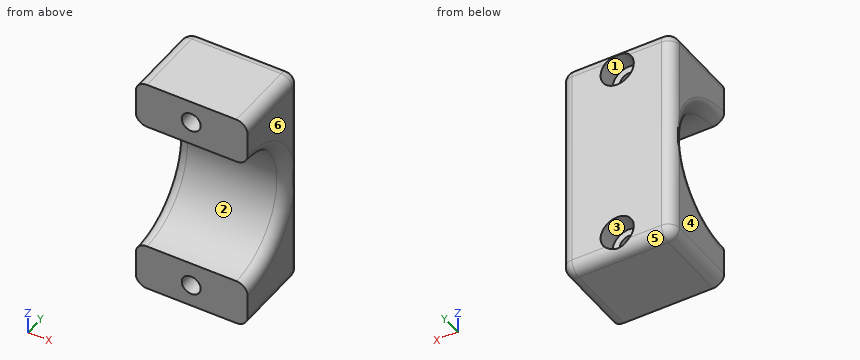
from build123d import *

# Parameters (mm, degrees)
SKETCH1_W                                      = 50.8
SKETCH1_H                                      = 19.05
BOSS_EXTRUDE1_DEPTH                            = 25.4
SKETCH2_R                                      = 14.9225
CUT_EXTRUDE1_DEPTH                             = 60.905780189
CBORE_FOR_6_BUTTON_HEAD_CAP_SCREW1_D           = 4.3053
CBORE_FOR_6_BUTTON_HEAD_CAP_SCREW1_CBORE_D     = 7.54126
CBORE_FOR_6_BUTTON_HEAD_CAP_SCREW1_CBORE_DEPTH = 4.3942
FILLET1_R                                      = 2.54


with BuildPart() as part:
    # Sketch1 → Boss-Extrude1 (new body)
    with BuildSketch(Plane(origin=(0, 0, 0), x_dir=(0, 0, -1), z_dir=(1, 0, 0))):
        with Locations((25.4, 9.525)):
            Rectangle(SKETCH1_W, SKETCH1_H)
    extrude(amount=BOSS_EXTRUDE1_DEPTH)

    # Sketch2 → Cut-Extrude1 (cut, through all)
    with BuildSketch(Plane(origin=(25.4, 0, 0), x_dir=(0, 0, -1), z_dir=(1, 0, 0))):
        with Locations((25.4, 0)):
            Circle(SKETCH2_R)
    extrude(amount=-CUT_EXTRUDE1_DEPTH, mode=Mode.SUBTRACT)

    # CBORE for #6 Button Head Cap Screw1 (through all)
    with Locations(Plane(origin=(0, 19.05, 0), x_dir=(1, 0, 0), z_dir=(0, 1, 0))):
        with Locations((12.594620829, 5.08), (12.594620829, 45.72)):
            CounterBoreHole(CBORE_FOR_6_BUTTON_HEAD_CAP_SCREW1_D / 2, CBORE_FOR_6_BUTTON_HEAD_CAP_SCREW1_CBORE_D / 2, CBORE_FOR_6_BUTTON_HEAD_CAP_SCREW1_CBORE_DEPTH)

    # Fillet1
    # the kernel refuses this fillet: 2.54 mm, written as the material it takes off along each edge
    with BuildSketch(Plane(origin=(22.86, 16.51, -48.26), x_dir=(0, 1, 0), z_dir=(1, 0, 0))) as fillet1_piece_1_section:
        Polygon((0, 0), (FILLET1_R, 0), (FILLET1_R, -FILLET1_R), (0, -FILLET1_R), align=None)
    fillet1_piece_1 = extrude(amount=FILLET1_R, mode=Mode.PRIVATE)
    fillet1_piece_1 = fillet1_piece_1 - Plane(origin=(22.86, 16.51, -48.26), x_dir=(0, -0.7071067811865475, 0.7071067811865475), z_dir=(1, 0, 0)) * Sphere(FILLET1_R, mode=Mode.PRIVATE)
    add(fillet1_piece_1, mode=Mode.SUBTRACT)
    with BuildSketch(Plane(origin=(22.86, 16.51, -2.54), x_dir=(1, 0, 0), z_dir=(0, 0, 1))) as fillet1_piece_2_section:
        Polygon((0, 0), (FILLET1_R, 0), (FILLET1_R, FILLET1_R), (0, FILLET1_R), align=None)
    fillet1_piece_2 = extrude(amount=FILLET1_R, mode=Mode.PRIVATE)
    fillet1_piece_2 = fillet1_piece_2 - Plane(origin=(22.86, 16.51, -2.54), x_dir=(-0.7071067811865475, -0.7071067811865475, 0), z_dir=(0, 0, 1)) * Sphere(FILLET1_R, mode=Mode.PRIVATE)
    add(fillet1_piece_2, mode=Mode.SUBTRACT)
    with BuildSketch(Plane(origin=(2.54, 16.51, -48.26), x_dir=(0, 1, 0), z_dir=(-1, 0, 0))) as fillet1_piece_3_section:
        Polygon((0, 0), (FILLET1_R, 0), (FILLET1_R, FILLET1_R), (0, FILLET1_R), align=None)
    fillet1_piece_3 = extrude(amount=FILLET1_R, mode=Mode.PRIVATE)
    fillet1_piece_3 = fillet1_piece_3 - Plane(origin=(2.54, 16.51, -48.26), x_dir=(0, -0.7071067811865475, 0.7071067811865475), z_dir=(-1, 0, 0)) * Sphere(FILLET1_R, mode=Mode.PRIVATE)
    add(fillet1_piece_3, mode=Mode.SUBTRACT)
    with BuildSketch(Plane(origin=(2.54, 16.51, -2.54), x_dir=(0, 0, 1), z_dir=(-1, 0, 0))) as fillet1_piece_4_section:
        Polygon((0, 0), (FILLET1_R, 0), (FILLET1_R, FILLET1_R), (0, FILLET1_R), align=None)
    fillet1_piece_4 = extrude(amount=FILLET1_R, mode=Mode.PRIVATE)
    fillet1_piece_4 = fillet1_piece_4 - Plane(origin=(2.54, 16.51, -2.54), x_dir=(0, -0.7071067811865475, -0.7071067811865475), z_dir=(-1, 0, 0)) * Sphere(FILLET1_R, mode=Mode.PRIVATE)
    add(fillet1_piece_4, mode=Mode.SUBTRACT)
    with BuildSketch(Plane(origin=(25.4, -6.35, -50.8), x_dir=(0, 0, 1), z_dir=(0, 1, 0))) as fillet1_piece_5:
        with BuildLine():
            CenterArc((FILLET1_R, -FILLET1_R), FILLET1_R, 90, 90)
            Line((0, -FILLET1_R), (0, 0))
            Line((0, 0), (FILLET1_R, 0))
        make_face()
    extrude(amount=22.86, mode=Mode.SUBTRACT)
    with BuildSketch(Plane(origin=(25.4, 19.05, -48.26), x_dir=(0, -1, 0), z_dir=(0, 0, 1))) as fillet1_piece_6:
        with BuildLine():
            CenterArc((FILLET1_R, -FILLET1_R), FILLET1_R, 90, 90)
            Line((0, -FILLET1_R), (0, 0))
            Line((0, 0), (FILLET1_R, 0))
        make_face()
    extrude(amount=45.72, mode=Mode.SUBTRACT)
    with BuildSketch(Plane(origin=(25.4, 0, -25.4), x_dir=(0, -0.413428527977308, -0.9105365738148667), z_dir=(0, -0.9105365738148667, 0.413428527977308))) as fillet1_piece_7:
        with BuildLine():
            CenterArc((14.9225 + FILLET1_R, -FILLET1_R), FILLET1_R, 90, 90)
            Line((14.9225 + FILLET1_R, 0), (14.9225, 0))
            Line((14.9225, 0), (14.9225, -FILLET1_R))
        make_face()
    revolve(axis=Axis((25.4, 0, -25.4), (1, 0, 0)), revolution_arc=228.840784647, mode=Mode.SUBTRACT)
    with BuildSketch(Plane(origin=(0, 0, -25.4), x_dir=(0, -0.413428527977308, -0.9105365738148667), z_dir=(0, -0.9105365738148667, 0.413428527977308))) as fillet1_piece_8:
        with BuildLine():
            CenterArc((14.9225 + FILLET1_R, FILLET1_R), FILLET1_R, 180, 90)
            Line((14.9225, FILLET1_R), (14.9225, 0))
            Line((14.9225, 0), (14.9225 + FILLET1_R, 0))
        make_face()
    revolve(axis=Axis((0, 0, -25.4), (1, 0, 0)), revolution_arc=228.840784647, mode=Mode.SUBTRACT)
    with BuildSketch(Plane(origin=(25.4, 16.51, 0), x_dir=(-1, 0, 0), z_dir=(0, -1, 0)), Plane(origin=(0, -6.35, -50.8), x_dir=(0, 0, 1), z_dir=(0, 1, 0)), Plane(origin=(0, 16.51, 0), x_dir=(0, 0, -1), z_dir=(0, -1, 0))) as fillet1_piece_9:
        with BuildLine():
            CenterArc((FILLET1_R, FILLET1_R), FILLET1_R, 180, 90)
            Line((0, FILLET1_R), (0, 0))
            Line((0, 0), (FILLET1_R, 0))
        make_face()
    extrude(amount=22.86, mode=Mode.SUBTRACT)
    with BuildSketch(Plane(origin=(0, 19.05, -48.26), x_dir=(0, -1, 0), z_dir=(0, 0, 1))) as fillet1_piece_10:
        with BuildLine():
            CenterArc((FILLET1_R, FILLET1_R), FILLET1_R, 180, 90)
            Line((0, FILLET1_R), (0, 0))
            Line((0, 0), (FILLET1_R, 0))
        make_face()
    extrude(amount=45.72, mode=Mode.SUBTRACT)
    with BuildSketch(Plane(origin=(2.54, 19.05, 0), x_dir=(0, -1, 0), z_dir=(1, 0, 0)), Plane(origin=(2.54, 19.05, -50.8), x_dir=(0, 0, 1), z_dir=(1, 0, 0))) as fillet1_piece_11:
        with BuildLine():
            CenterArc((FILLET1_R, FILLET1_R), FILLET1_R, 180, 90)
            Line((0, FILLET1_R), (0, 0))
            Line((0, 0), (FILLET1_R, 0))
        make_face()
    extrude(amount=20.32, mode=Mode.SUBTRACT)


solid = part.part
Geometry check sheet. Reference: the model listing, model coordinates, mm. Face numbers are marked on the shaded views. A direction names the side the tool comes from. Round coordinates to 2 decimals unless told otherwise and drop trailing zeros. Loops run counter-clockwise (first coordinate to the right, second up) from the corner with the lowest first, then second, coordinate; pieces in that order, holes last. Notation, with made-up numbers: (34, -13) -> (41, -13) arc R23 cw to (41, 13) -> close; hole circle Ø1 at (41, 33). An arc over 180 degrees is marked (long way). Answer as a JSON object with one key per item and string values. Group by question number.
Item 1: Cross-section at C-C, the plane x = 12. Count the separate pieces of the cut face and the enclosed holes in it, plus the area to 3 significant figures.
Item 2: Release check for a two-part mould opening along X. For the marked faces 3, 4, 5 and 6 record: pulls with the +X half, pulls with the -X half, needs draft (parallel to the pull), parting line crosses it, or undercut.
Item 3: Cross-section at A-A, the plane z = -5.08. Record the cut outline in (x, y), plus the area to 3 significant figures.
Item 4: Depth check by flat-ended pin: pin 1 Ø4 at (x, z) = (13, -44.5) entering from +Y; pin 2 Ø4 at (x, z) = (12.59, -5.08) entering from -Y; pin 3 Ø1 at (y, z) = (8.5, -13.5) entering from -X; pin 4 Ø8 at (x, z) = (11.5, -19) entering from -Y. Enter the tip coordinate at first touch or a pass-through.
Item 5: Set-up check for the marked faces 1 and 2: record each of +Z, -Z, +X, -X, +Y, -Y from which the full face is reachable in a straight line by a thin tool's end or side.
Item 6: Thickness scan on line 1 along Z through (x, y) = (11, 9.25); line 2 along X through (y, z) = (6, -45.72); line 3 along Z through (x, y) = (10.75, 3). Record the ranges inside material, lowest first.
Determined:
{
 "1": {"separate pieces": "3", "enclosed holes": "0", "area": "429 mm²"},
 "2": {"face 3": "undercut", "face 4": "pulls with the -X half", "face 5": "needs draft", "face 6": "pulls with the +X half"},
 "3": {"outline": "(0, 0) -> (10.44, 0) -> (10.44, 14.66) -> (8.82, 14.66) -> (8.82, 19.05) -> (2.54, 19.05) arc R2.54 ccw to (0, 16.51) -> close; (14.75, 0) -> (25.4, 0) -> (25.4, 16.51) arc R2.54 ccw to (22.86, 19.05) -> (16.37, 19.05) -> (16.37, 14.66) -> (14.75, 14.66) -> close", "area": "385 mm²"},
 "4": {"pin 1": "stops at y = 14.66", "pin 2": "passes through", "pin 3": "stops at x = 1.55", "pin 4": "stops at y = 10.7"},
 "5": {"face 1": "+Y", "face 2": "+X, -X, -Y"},
 "6": {"line 1": "z = -50.8 to -47.17, -44.27 to -37.11, -13.69 to -6.53, -3.63 to 0", "line 2": "x = 0 to 10.44, 14.75 to 25.4", "line 3": "z = -50.8 to -46.83, -44.61 to -40.02, -10.78 to -6.19, -3.97 to 0"}
}
